Part model, mm, in its own coordinate system. Coordinates: 2 decimals unless noted, no trailing zeros. Write each loop counter-clockwise with the first axis right and the second up, starting at its lowest first coordinate (ties: lowest second). Pieces come first, ordered by that corner, then holes. Notation, with made-up numbers: (62, -6) -> (110, -6) arc R4 cw to (110, 1) -> close; hole circle Ø1 at (40.25, -28.5). An arc over 180 degrees is marked (long way). Write item = value, one per line. Start each with the question number.
Q1. Pin check, flat tips, straight feed: P1, Ø1, axis at x = 109.5, y = -8.5, coming from the -Z side; P2, Ø0.7, axis at x = -63, z = 0, coming from the +Y side. Stop position of each tip, or through.
Q2. Band-saw the part on A-A, the plane x = 86.5. List the corners of the cut face in (y, z), plus the area to 3 significant figures.
Q3. Band-saw the part on C-C, the plane y = 4.25. List the corners of the cut face in (x, z).
Q4. Band-saw the part on B-B, the plane y = -8. List the corners of the cut face in (x, z), plus the area to 3 significant figures.
Q5. Probe line 1 (Y direction, x = 52, z = -9.75); line 2 (Y direction, x = 85, z = -1.25); line 3 (Z direction, x = -5.5, y = -0.25). List the from-to ranges inside material, lowest first.
from build123d import *

# Parameters (mm, degrees)
BOSS_EXTRUDE1_DEPTH      = 150
BOSS_EXTRUDE1_DEPTH_BACK = 150
SKETCH1_R                = 12
CUT_EXTRUDE1_DEPTH       = 151.956947505
LPATTERN1_COUNT          = 20
LPATTERN1_PITCH          = 6.283185307


with BuildPart() as part:
    # Sketch1 → Boss-Extrude1 (new, two sides: drawn at the far end of the back side and taken through both)
    with BuildSketch(Plane(origin=(0, 0, 0), x_dir=(0, 0, -1), z_dir=(1, 0, 0)).offset(-BOSS_EXTRUDE1_DEPTH_BACK)):
        Circle(SKETCH1_R)
    extrude(amount=BOSS_EXTRUDE1_DEPTH + BOSS_EXTRUDE1_DEPTH_BACK)

    # Sketch2 → Cut-Extrude1 (cut, symmetric)
    with BuildSketch(Plane.XY):
        Polygon((-62.170982331, 7.5), (-63.492723813, 7.5), (-65.130589867, 12), (-60.533116276, 12), align=None)
    cut_extrude1 = extrude(amount=CUT_EXTRUDE1_DEPTH, both=True, mode=Mode.SUBTRACT)

    # LPattern1: Cut-Extrude1 ×20
    with Locations(*[(i * LPATTERN1_PITCH, 0, 0) for i in range(1, LPATTERN1_COUNT)]):
        add(cut_extrude1, mode=Mode.SUBTRACT)


solid = part.part
Ans:
q1.P1 = -8.94
q1.P2 = 7.5
q2.outline = circle Ø24 at (0, 0)
q2.area = 452 mm2
q3.outline = (-150, -11.22) -> (150, -11.22) -> (150, 11.22) -> (-150, 11.22) -> close
q4.outline = (-150, -8.94) -> (150, -8.94) -> (150, 8.94) -> (-150, 8.94) -> close
q4.area = 5,370 mm2
q5.line_1 = -7 to 7
q5.line_2 = -11.93 to 11.93
q5.line_3 = -12 to 12
